The figure shows three views and two pictorial views of one solid part (mm, origin at its lowest corner). Answer the questions. Coordinates: 2 decimals unless noted, no trailing zeros. Order: outer loops, then holes, each group sorted by start corner. A loop starts at its lowest first (then second) coordinate and runs counter-clockwise, first axis right, second up.
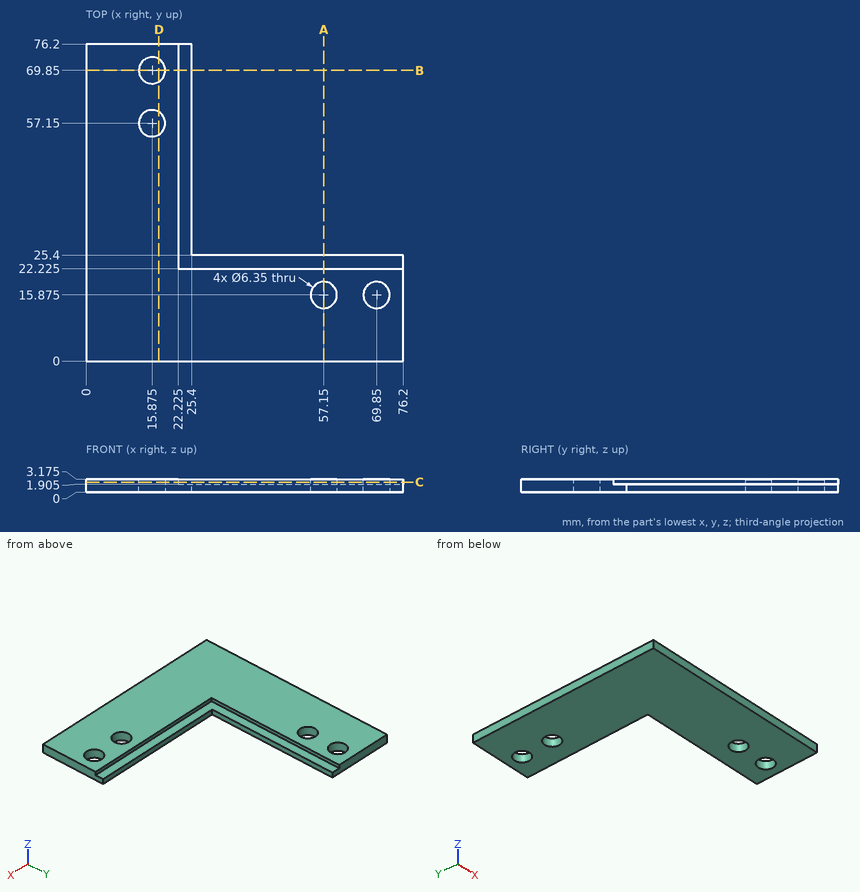
Q1. The part is cut by section D-D, the plane x = 17.5. Determine the outline of the cut face in (y, z) (3 decimals), then the cut area to 3 significant figures.
Q2. The part is cut by section C-C, the plane z = 2.4. Determine the outline of the cut face in (x, y) (3 decimals).
Q3. Straight lines are drawn through the part: L1, parallel to Y at x = 69.85, z = 1.1; L2, parallel to Y at x = 57.15, z = 2.2 (3 decimals). For each, find the intervals that lie inside material, in ascending order.
Q4. The part is cut by section A-A, the plane x = 57.15. Determine the outline of the cut face in (y, z) (3 decimals).
Q5. Each of these flat-tipped pins is pushed along its axis until it touches: P1, Ø0.6, axis at y = 59.5, z = 1, coming from the +X side; P2, Ø0.6, axis at x = 60, z = 2.5, coming from the +Y side (3 decimals); P3, Ø0.6, axis at x = 61.5, z = 1, coming from the +Y side. Where does it stop, or does it pass through?
Computed values:
1. outline: (0, 0) - (54.422, 0) - (54.422, 3.175) - (0, 3.175) - close; (59.878, 0) - (67.122, 0) - (67.122, 3.175) - (59.878, 3.175) - close; (72.578, 0) - (76.2, 0) - (76.2, 3.175) - (72.578, 3.175) - close
1. area: 207 mm2
2. outline: (0, 0) - (76.2, 0) - (76.2, 22.225) - (22.225, 22.225) - (22.225, 76.2) - (0, 76.2) - close; hole circle Ø6.35 at (15.875, 57.15); hole circle Ø6.35 at (15.875, 69.85); hole circle Ø6.35 at (57.15, 15.875); hole circle Ø6.35 at (69.85, 15.875)
3. L1: y = 0 to 12.7, 19.05 to 25.4
3. L2: y = 0 to 12.7, 19.05 to 22.225
4. outline: (0, 0) - (12.7, 0) - (12.7, 3.175) - (0, 3.175) - close; (19.05, 0) - (25.4, 0) - (25.4, 1.905) - (22.225, 1.905) - (22.225, 3.175) - (19.05, 3.175) - close
5. P1: stops at x = 25.4
5. P2: stops at y = 22.225
5. P3: stops at y = 25.4
